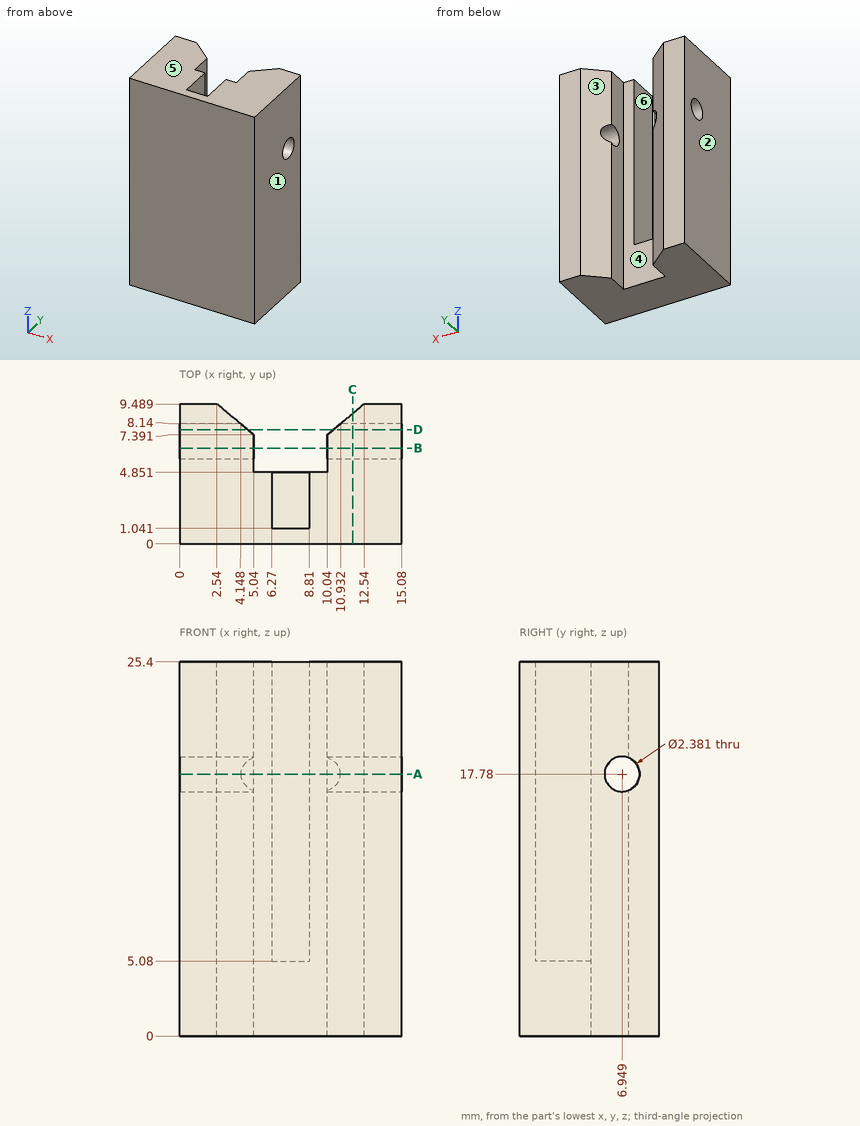
For this review, use the dimensioned drawing (mm, ordinates from the lowest corner) and the shaded views. A direction names the side the tool comes from. Coordinates: 2 decimals unless noted, no trailing zeros. Write each loop counter-clockwise with the first axis right and the second up, starting at its lowest first coordinate (ties: lowest second). Pieces come first, ordered by that corner, then holes. Notation, with made-up numbers: (39, 12) - (58, 12) arc R14 cw to (58, 23) - close; hole circle Ø2 at (73.25, -23). An arc over 180 degrees is marked (long way). Answer in a Markdown table with one row per item. Add a question column.
Q1. Draft analysis for pull direction X (two halves, no side actions). For the marked faces 1, 2 and 3, state which applies: +X half, -X half, draft (parallel to the pull), parting line (faces both ways), or undercut.
Q2. To check wall thickness, follow line 1 along X through (y, z) = (3.25, 9.75); line 2 along Y through (x, z) = (1.25, 17.78); line 3 along X through (y, z) = (6, 2.25). State the ranges of each line that lie inside material, in increasing order. Write a range as from..to.
Q3. For the marked faces 4, 5 and 6, list the 3-axis set-ups (+Z, -Z, +X, -X, +Y, -Y) from which the entire face can be reached by the end or side of a thin tool; tool diameter is ignored.
Q4. Consider section C-C on x = 11.75. Give the boundary of the cut face in (y, z), then the cut area to 3 significant figures.
Q5. Consider section A-A on z = 17.78. Give the boundary of the cut face in (x, y).
Q6. Clearance check with flat-ended pins moving along their axes: pin 1 (3 mm diameter, centred on x = 8, y = 4, fed in from +Z); pin 2 (6 mm diameter, centred on x = 8, z = 19.5, fed in from +Y); pin 3 (2 mm diameter, centred on y = 6.95, z = 17.78, fed in from +X); pin 4 (1.5 mm diameter, centred on x = 11.5, z = 20, fed in from +Y) (1 decimal). State where each tip first meets the part, or that it passes through.
Q7. Consider section D-D on y = 7.75. Give the boundary of the cut face in (x, z).
Q8. Consider section B-B on y = 6.5. Give the boundary of the cut face in (x, z), then the cut area to 3 significant figures.
Answers below:
| question | item | result |
|---|---|---|
| 1 | face 1 | +X half |
| 1 | face 2 | -X half |
| 1 | face 3 | undercut |
| 2 | line 1 | 0..6.27, 8.81..15.08 |
| 2 | line 2 | 0..5.76, 8.14..9.49 |
| 2 | line 3 | 0..5.04, 10.04..15.08 |
| 3 | face 4 | +Z, -Z, +Y |
| 3 | face 5 | +Z, +X, -X, +Y, -Y |
| 3 | face 6 | +Z, +Y |
| 4 | outline | (0, 0) - (8.83, 0) - (8.83, 25.4) - (0, 25.4) - close; hole circle Ø2.38 at (6.95, 17.78) |
| 4 | area | 220 mm² |
| 5 | outline | (0, 0) - (15.08, 0) - (15.08, 5.76) - (10.04, 5.76) - (10.04, 4.85) - (8.81, 4.85) - (8.81, 1.04) - (6.27, 1.04) - (6.27, 4.85) - (5.04, 4.85) - (5.04, 5.76) - (0, 5.76) - close; (0, 8.14) - (4.15, 8.14) - (2.54, 9.49) - (0, 9.49) - close; (10.93, 8.14) - (15.08, 8.14) - (15.08, 9.49) - (12.54, 9.49) - close |
| 6 | pin 1 | z = 25.4 |
| 6 | pin 2 | y = 8.2 |
| 6 | pin 3 | through |
| 6 | pin 4 | y = 9.2 |
| 7 | outline | (0, 0) - (4.61, 0) - (4.61, 16.9) - (0, 16.9) - close; (0, 18.66) - (4.61, 18.66) - (4.61, 25.4) - (0, 25.4) - close; (10.47, 0) - (15.08, 0) - (15.08, 16.9) - (10.47, 16.9) - close; (10.47, 18.66) - (15.08, 18.66) - (15.08, 25.4) - (10.47, 25.4) - close |
| 8 | outline | (0, 0) - (5.04, 0) - (5.04, 16.68) - (0, 16.68) - close; (0, 18.88) - (5.04, 18.88) - (5.04, 25.4) - (0, 25.4) - close; (10.04, 0) - (15.08, 0) - (15.08, 16.68) - (10.04, 16.68) - close; (10.04, 18.88) - (15.08, 18.88) - (15.08, 25.4) - (10.04, 25.4) - close |
| 8 | area | 234 mm² |
